from build123d import *

# Parameters (mm, degrees)
CUT_EXTRUDE1_DEPTH      = 1
CUT_EXTRUDE1_DEPTH_BACK = 23


with BuildPart() as part:
    # Sketch1 → Revolve1 (revolve)
    with BuildSketch(Plane.XY):
        Polygon((-6.562817936, 5), (-6.562817936, 20), (-4.062817936, 20), (-2.242966765, 15), (1.117330893, 15), (2.937182064, 20), (5.437182064, 20), (5.437182064, 14), (15.437182064, 14), (15.437182064, 5), align=None)
    revolve(axis=Axis((-16.510808735, 0, 0), (1, 0, 0)))

    # Sketch2 → Cut-Extrude1 (cut, two sides)
    with BuildSketch(Plane(origin=(15.437182064, 0, 0), x_dir=(0, 0, -1), z_dir=(1, 0, 0))) as cut_extrude1_sk:
        with BuildLine():
            Line((4.769696007, -1.5), (6.4, -1.5))
            Line((6.4, -1.5), (6.4, 1.5))
            Line((6.4, 1.5), (4.769696007, 1.5))
            ThreePointArc((4.769696007, 1.5), (5, 0), (4.769696007, -1.5))
        make_face()
    extrude(amount=CUT_EXTRUDE1_DEPTH, mode=Mode.SUBTRACT)
    extrude(cut_extrude1_sk.sketch, amount=-CUT_EXTRUDE1_DEPTH_BACK, mode=Mode.SUBTRACT)


solid = part.part
Work out the finished part from the listing and answer in its coordinate system (mm). A direction names the side the tool comes from. Give positions to 0.01 mm unless a question says otherwise; leave off trailing zeros. Loops run counter-clockwise (first coordinate to the right, second up) from the corner with the lowest first, then second, coordinate; pieces in that order, holes last. Notation, with made-up numbers: (28, 50) -> (67, 50) arc R37 cw to (67, 87) -> close; hole circle Ø10 at (18.25, 47). An arc over 180 degrees is marked (long way). Use a Markdown table: item, result. Add a question column.
1) Consider line 1 along Z through (x, y) = (3.75, 0); line 2 along Z through (x, y) = (9.25, 0); line 3 along X through (y, z) = (-9.5, 15). Determine where each line is inside the solid, lowest interval first.
2) Each of these flat-tipped pins is pushed along its axis until it touches: P1, Ø2, axis at x = 5.5, z = 8.5, coming from the -Y side; P2, Ø0.8, axis at x = 10, z = -5.5, coming from the +Y side; P3, Ø12, axis at x = -3.5, y = 16, coming from the -Z side. Where does it stop, or does it pass through?
3) The part is cut by section D-D, the plane x = 4.5. Determine the outline of the cut face in (y, z), plus the area to 3 significant figures.
4) The part is cut by section C-C, the plane y = 0. Determine the outline of the cut face in (x, z).
5) The part is cut by section B-B, the plane x = 8.5. Determine the outline of the cut face in (y, z), plus the area to 3 significant figures.
6) Which of the six approach directions +Z, -Z, +X, -X, +Y, -Y give full straight-line access (tool end or side, diameter ignored) to faces 4 (the flat face through (5, -1.5, -6)), 5 (the conical face through (-2.33, 14.54, 4.58)), 6 (the flat face through (5.437, 4, 14)), 7 (the flat face through (-6.563, -4, -4))?
7) The part is cut by section A-A, the plane z = 0. Determine the outline of the cut face in (x, y), plus the area to 3 significant figures.
8) For a pull along Y with two mould halves and no side action, classify faces 1 (the flat face through (15.437, 6, 0)), 2 (the cylindrical face through (10.507, 12.932, -5.362)), 3 (the flat face through (5, 0, -6.4)) as +Y half, -Y half, draft (parallel to the pull), parting line (faces both ways), or undercut.
Reported:
| question | item | result |
|---|---|---|
| 1 | line 1 | z = -20 to -6.4, 5 to 20 |
| 1 | line 2 | z = -14 to -6.4, 5 to 14 |
| 1 | line 3 | x = -6.56 to -3.25, 2.12 to 5.44 |
| 2 | P1 | stops at y = -18.54 |
| 2 | P2 | stops at y = 13.04 |
| 2 | P3 | stops at z = -17.31 |
| 3 | outline | circle Ø40 at (0, 0); hole (-1.5, -6.4) -> (1.5, -6.4) -> (1.5, -4.77) arc R5 ccw (long way) to (-1.5, -4.77) -> close |
| 3 | area | 1,170 mm^2 |
| 4 | outline | (-6.56, -20) -> (-4.06, -20) -> (-2.24, -15) -> (1.12, -15) -> (2.94, -20) -> (5.44, -20) -> (5.44, -14) -> (15.44, -14) -> (15.44, -6.4) -> (-6.56, -6.4) -> close; (-6.56, 5) -> (15.44, 5) -> (15.44, 14) -> (5.44, 14) -> (5.44, 20) -> (2.94, 20) -> (1.12, 15) -> (-2.24, 15) -> (-4.06, 20) -> (-6.56, 20) -> close |
| 5 | outline | circle Ø28 at (0, 0); hole (-1.5, -6.4) -> (1.5, -6.4) -> (1.5, -4.77) arc R5 ccw (long way) to (-1.5, -4.77) -> close |
| 5 | area | 533 mm^2 |
| 6 | face 4 | +X, -X |
| 6 | face 5 | none |
| 6 | face 6 | +X |
| 6 | face 7 | +Z, -Z, -X, +Y, -Y |
| 7 | outline | (-6.56, -20) -> (-4.06, -20) -> (-2.24, -15) -> (1.12, -15) -> (2.94, -20) -> (5.44, -20) -> (5.44, -14) -> (15.44, -14) -> (15.44, -5) -> (-6.56, -5) -> close; (-6.56, 5) -> (15.44, 5) -> (15.44, 14) -> (5.44, 14) -> (5.44, 20) -> (2.94, 20) -> (1.12, 15) -> (-2.24, 15) -> (-4.06, 20) -> (-6.56, 20) -> close |
| 7 | area | 488 mm^2 |
| 8 | face 1 | draft |
| 8 | face 2 | parting line |
| 8 | face 3 | undercut |
